The model under review builds one solid part; all positions refer to its coordinate system, in mm. A direction names the side the tool comes from. Give positions to 0.01 mm unless a question says otherwise; leave off trailing zeros. Order: outer loops, then holes, each group sorted by start corner. A loop starts at its lowest first (then second) coordinate and runs counter-clockwise, first axis right, second up. Notation, with made-up numbers: M 72,65 L 106,65 A30 cw 106,103 Z; hole C -9,-18 d2. An arc over 180 degrees is marked long. One line per question, with ' | ' between items. Start each with the question number.
1. We need section D-D on y = 6. Write out the cut boundary in (x, z), then the cut area to 3 significant figures.
2. We need section B-B on x = 10. Write out the cut boundary in (y, z).
3. Wall thickness on L1, parallel to Z at x = -21, y = -12; L2, parallel to X at y = 0, z = 5; L3, parallel to Z at x = -5.5, y = 6: over which ranges is each line inside the solid? List them lowest first.
4. The part is to be moulded in two halves that separate along Z. For faces 1 (the face through (5, 6, 58)), 2 (the face through (5, -19, 9)), 3 (the face through (5, 6, 14)), say which applies: +Z half, -Z half, draft (parallel to the pull), parting line (faces both ways), or undercut.
5. For faces 4 (the face through (5, 6, 0)), 5 (the face through (-18, -1, 11)), list the 3-axis set-ups (+Z, -Z, +X, -X, +Y, -Y) from which the entire face can be reached by the end or side of a thin tool; tool diameter is ignored.
6. Insertion check: P1, Ø1.8, axis at y = 4, z = 48, coming from the -X side; P2, Ø6, axis at y = -4, z = 44, coming from the +X side; P3, Ø8, axis at y = -7, z = 36, coming from the -X side. Each pin has a flat end and moves straight along its axis. Give the tip position at first contact, or say it passes through.
7. We need section C-C on x = 0. Write out the cut boundary in (y, z).
8. We need section A-A on z = 29. Write out the cut boundary in (x, y), then the cut area to 3 significant figures.
```python
from build123d import *

# Parameters (mm, degrees)
SKETCH1_R                = 7.5
BOSS_EXTRUDE1_DEPTH      = 58
SKETCH5_R                = 7
CUT_EXTRUDE1_DEPTH       = 81
CUT_EXTRUDE3_DEPTH       = 22.0000001
CUT_EXTRUDE3_DEPTH_BACK  = 20
SKETCH7_W                = 16
SKETCH7_H                = 6
CUT_EXTRUDE5_DEPTH       = 22
CUT_EXTRUDE5_DEPTH_BACK  = 20
CUT_EXTRUDE14_DEPTH      = 24
CUT_EXTRUDE14_DEPTH_BACK = 24


with BuildPart() as part:
    # Sketch1 → Boss-Extrude1 (new body)
    with BuildSketch(Plane.XY):
        with BuildLine():
            Line((-34, -19), (31, -19))
            Line((31, -19), (46, -10.339745962))
            Line((46, -10.339745962), (46, 12.339745962))
            Line((46, 12.339745962), (31, 21))
            Line((31, 21), (2.66060556, 21))
            ThreePointArc((2.66060556, 21), (-17.33939444, 16.82575695), (-34, 5))
            Line((-34, 5), (-34, -19))
        make_face()
        Circle(SKETCH1_R, mode=Mode.SUBTRACT)
    extrude(amount=BOSS_EXTRUDE1_DEPTH)

    # Sketch5 → Cut-Extrude1 (cut, through all)
    with BuildSketch(Plane(origin=(46, 0, 0), x_dir=(0, 0, -1), z_dir=(1, 0, 0))):
        with Locations((-29, 1)):
            Circle(SKETCH5_R)
    extrude(amount=-CUT_EXTRUDE1_DEPTH, mode=Mode.SUBTRACT)

    # Sketch6 → Cut-Extrude3 (cut, two sides)
    with BuildSketch(Plane(origin=(0, 0, 0), x_dir=(1, 0, 0), z_dir=(0, 1, 0))) as cut_extrude3_sk:
        Polygon((-226.60339564, -14), (-34, -14), (20, -14), (20, -44), (-34, -44), (-226.60339564, -44), (-611.81018692, -44), (-611.81018692, -14), align=None)
    extrude(amount=CUT_EXTRUDE3_DEPTH, mode=Mode.SUBTRACT)
    extrude(cut_extrude3_sk.sketch, amount=-CUT_EXTRUDE3_DEPTH_BACK, mode=Mode.SUBTRACT)

    # Sketch7 → Cut-Extrude5 (cut, two sides)
    with BuildSketch(Plane(origin=(0, 0, 0), x_dir=(1, 0, 0), z_dir=(0, 1, 0))) as cut_extrude5_sk:
        with Locations((-26, -11)):
            Rectangle(SKETCH7_W, SKETCH7_H)
        with Locations((-26, -47)):
            Rectangle(SKETCH7_W, SKETCH7_H)
    extrude(amount=CUT_EXTRUDE5_DEPTH, mode=Mode.SUBTRACT)
    extrude(cut_extrude5_sk.sketch, amount=-CUT_EXTRUDE5_DEPTH_BACK, mode=Mode.SUBTRACT)

    # Sketch14 → Cut-Extrude14 (cut, two sides)
    with BuildSketch(Plane(origin=(0, 0, 0), x_dir=(1, 0, 0), z_dir=(0, 1, 0))) as cut_extrude14_sk:
        Polygon((31, 0), (46, 0), (46, -15), align=None)
        Polygon((31, -58), (46, -58), (46, -43), align=None)
    extrude(amount=CUT_EXTRUDE14_DEPTH, mode=Mode.SUBTRACT)
    extrude(cut_extrude14_sk.sketch, amount=-CUT_EXTRUDE14_DEPTH_BACK, mode=Mode.SUBTRACT)


solid = part.part
```
Entries:
1) outline: M -33.05,0 L -4.5,0 L -4.5,14 L -18,14 L -18,8 L -33.05,8 Z; M -33.05,50 L -18,50 L -18,44 L -4.5,44 L -4.5,58 L -33.05,58 Z; M 4.5,0 L 31,0 L 46,15 L 46,24.1 L 20,24.1 L 20,14 L 4.5,14 Z; M 4.5,44 L 20,44 L 20,33.9 L 46,33.9 L 46,43 L 31,58 L 4.5,58 Z | area: 2,080 mm^2
2) outline: M -19,0 L 21,0 L 21,14 L -19,14 Z; M -19,44 L 21,44 L 21,58 L -19,58 Z
3) L1: z = 0 to 8, 50 to 58 | L2: x = -34 to -7.5, 7.5 to 36 | L3: z = 0 to 14, 44 to 58
4) face 1: +Z half | face 2: draft | face 3: undercut
5) face 4: -Z, +X, -X, +Y, -Y | face 5: -X, +Y, -Y
6) P1: stops at x = -18 | P2: stops at x = 46 | P3: stops at x = 20
7) outline: M -19,0 L -7.5,0 L -7.5,14 L -19,14 Z; M -19,44 L -7.5,44 L -7.5,58 L -19,58 Z; M 7.5,0 L 20.93,0 L 20.93,14 L 7.5,14 Z; M 7.5,44 L 20.93,44 L 20.93,58 L 7.5,58 Z
8) outline: M 20,-19 L 31,-19 L 46,-10.34 L 46,-6 L 20,-6 Z; M 20,8 L 46,8 L 46,12.34 L 31,21 L 20,21 Z | area: 546 mm^2
